Study the drawing (mm; zero at the part's minimum x, y, z) and answer. A direction names the side the tool comes from. Coordinates: 2 decimals unless noted, no trailing zeros. Write each loop counter-clockwise with the first axis right and the second up, starting at its lowest first coordinate (ties: lowest second). Pieces come first, ordered by that corner, then holes. Notation, with made-up numbers: (1.25, -39.75) -> (26.25, -39.75) arc R35 ccw to (26.25, -4.75) -> close; hole circle Ø10 at (-24, -29.5). An arc over 180 degrees is marked (long way). Answer in a Markdown table with one row per item. Add a question column.
Item 1: Section A-A on y = 4.25 is taken. Write down the section's boundary in (x, z), then the cut area to 3 significant figures.
Item 2: Section C-C on z = 1.8 is taken. Write down the section's boundary in (x, y), then the cut area to 3 significant figures.
Item 3: Given pin 1 Ø0.5 at (y, z) = (5.5, 0.5) entering from -X; pin 2 Ø0.5 at (y, z) = (5.5, 0.5) entering from +X; pin 3 Ø1 at (x, z) = (11.5, 1.5) entering from -Y; pin 4 Ø1.5 at (x, y) = (3, 4.25) entering from +Z, each flat-ended and moving along its own axis, determine where each tip first touches the part or whether it passes through.
Item 4: Straight lines are drawn through the part: line 1 (X direction, y = 4.25, z = 0.75); line 2 (X direction, y = 1.55, z = 1.4); line 3 (X direction, y = 4.8, z = 0.55). For each, find the intervals that lie inside material, in ascending order. Write a range as from..to.
Item 5: For a pull along X with two mould halves and no side action, classify the marked faces 3, 4, 5 and 6 as +X half, -X half, draft (parallel to the pull), parting line (faces both ways), or undercut.
Item 6: Which of the six approach directions +Z, -Z, +X, -X, +Y, -Y give full straight-line access (tool end or side, diameter ignored) to the marked faces 1 and 2?
Item 7: Section D-D on x = 3 is taken. Write down the section's boundary in (y, z).
Item 8: Section B-B on y = 0.65 is taken. Write down the section's boundary in (x, z), then the cut area to 3 significant figures.
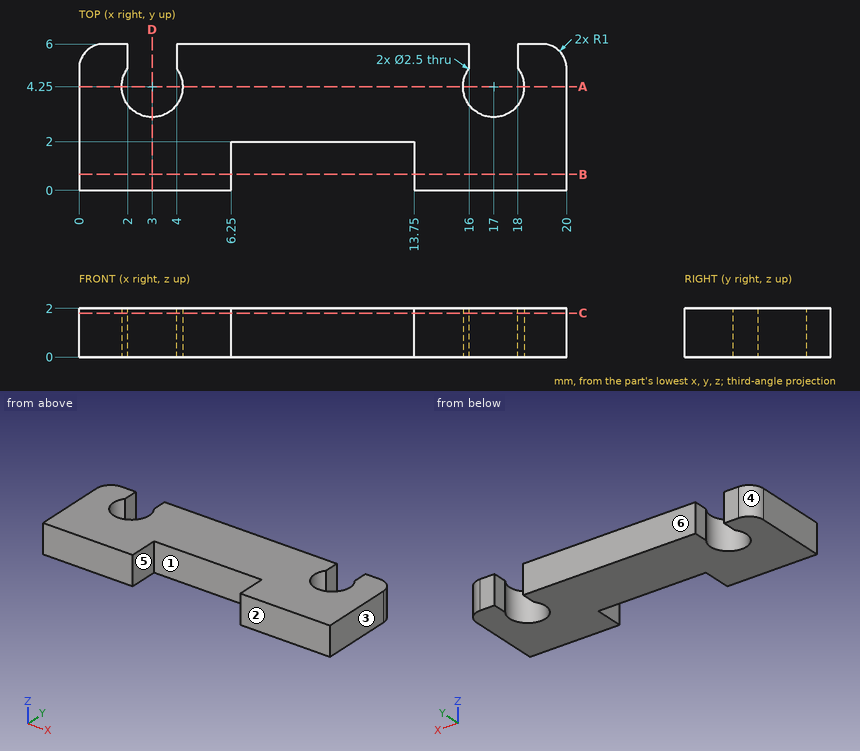
Results below:
| question | item | result |
|---|---|---|
| 1 | outline | (0, 0) -> (1.75, 0) -> (1.75, 2) -> (0, 2) -> close; (4.25, 0) -> (15.75, 0) -> (15.75, 2) -> (4.25, 2) -> close; (18.25, 0) -> (20, 0) -> (20, 2) -> (18.25, 2) -> close |
| 1 | area | 30.0 mm2 |
| 2 | outline | (0, 0) -> (6.25, 0) -> (6.25, 2) -> (13.75, 2) -> (13.75, 0) -> (20, 0) -> (20, 5) arc R1 ccw to (19, 6) -> (18, 6) -> (18, 5) arc R1.25 cw (long way) to (16, 5) -> (16, 6) -> (4, 6) -> (4, 5) arc R1.25 cw (long way) to (2, 5) -> (2, 6) -> (1, 6) arc R1 ccw to (0, 5) -> close |
| 2 | area | 92.2 mm2 |
| 3 | pin 1 | stops at x = 0.03 |
| 3 | pin 2 | stops at x = 19.97 |
| 3 | pin 3 | stops at y = 2 |
| 3 | pin 4 | passes through |
| 4 | line 1 | x = 0..1.75, 4.25..15.75, 18.25..20 |
| 4 | line 2 | x = 0..6.25, 13.75..20 |
| 4 | line 3 | x = 0..1.88, 4.12..15.88, 18.12..20 |
| 5 | face 3 | +X half |
| 5 | face 4 | -X half |
| 5 | face 5 | undercut |
| 5 | face 6 | draft |
| 6 | face 1 | +Z, -Z, -Y |
| 6 | face 2 | +Z, -Z, +X, -X, -Y |
| 7 | outline | (0, 0) -> (3, 0) -> (3, 2) -> (0, 2) -> close |
| 8 | outline | (0, 0) -> (6.25, 0) -> (6.25, 2) -> (0, 2) -> close; (13.75, 0) -> (20, 0) -> (20, 2) -> (13.75, 2) -> close |
| 8 | area | 25.0 mm2 |
